Could you check a few things on this model? Use its own coordinates, in mm. A direction names the side the tool comes from. Give positions to 0.01 mm unless a question says otherwise; leave off trailing zeros. Loops run counter-clockwise (first coordinate to the right, second up) from the corner with the lowest first, then second, coordinate; pieces in that order, holes last. Notation, with made-up numbers: (1, 73) - (37, 73) arc R25 cw to (37, 99) - close; hole circle Ø8 at (6.25, 81.25). An arc over 180 degrees is marked (long way). Write each question's results on one line, items separated by ' | '. Start each with the question number.
```python
from build123d import *

# Parameters (mm, degrees)
SKETCH1_R             = 37.5
BOSS_EXTRUDE1_DEPTH   = 10
SKETCH2_R             = 31.5
CUT_EXTRUDE1_DEPTH    = 6.5
SKETCH4_R             = 15.75
BOSS_EXTRUDE2_DEPTH   = 6.5
SKETCH5_R             = 3
CUT_EXTRUDE2_DEPTH    = 3.5
CIRPATTERN3_OUTLINE_R = 3
CIRPATTERN3_DEPTH     = 3.5
BOSS_EXTRUDE3_DEPTH   = 5
CIRPATTERN4_COUNT     = 4
SKETCH9_R             = 4.5
CUT_EXTRUDE3_DEPTH    = 2
CIRPATTERN5_COUNT     = 4
SKETCH10_R            = 1
CUT_EXTRUDE4_DEPTH    = 5
LPATTERN1_COUNT       = 2
LPATTERN1_PITCH       = 174
LPATTERN1_COUNT_DIR2  = 2
LPATTERN1_PITCH_DIR2  = 24
SKETCH11_R            = 2
CUT_EXTRUDE5_DEPTH    = 1
LPATTERN2_COUNT       = 2
LPATTERN2_PITCH       = 174
LPATTERN2_COUNT_DIR2  = 2
LPATTERN2_PITCH_DIR2  = 24


# Read off the part's stored shape, not the designer's step: CirPattern3
with BuildPart() as part:
    # Sketch1 → Boss-Extrude1 (new body)
    with BuildSketch(Plane(origin=(0, 0, 0), x_dir=(1, 0, 0), z_dir=(0, 1, 0))):
        with Locations(Location((0, 0, 0), (0, 0, 270))):
            Circle(SKETCH1_R)
    extrude(amount=BOSS_EXTRUDE1_DEPTH)

    # Sketch2 → Cut-Extrude1 (cut)
    with BuildSketch(Plane(origin=(0, 10, 0), x_dir=(1, 0, 0), z_dir=(0, 1, 0))):
        with Locations(Location((0, 0, 0), (0, 0, 270))):
            Circle(SKETCH2_R)
    extrude(amount=-CUT_EXTRUDE1_DEPTH, mode=Mode.SUBTRACT)

    # Sketch4 → Boss-Extrude2 (add)
    with BuildSketch(Plane(origin=(0, 3.5, 0), x_dir=(1, 0, 0), z_dir=(0, 1, 0))):
        with Locations(Location((0, 0, 0), (0, 0, 90))):
            Circle(SKETCH4_R)
    extrude(amount=BOSS_EXTRUDE2_DEPTH)

    # Sketch5 → Cut-Extrude2 (cut)
    with BuildSketch(Plane.XZ):
        with Locations(Location((0, 25, 0), (0, 0, 270))):
            Circle(SKETCH5_R)
    extrude(amount=-CUT_EXTRUDE2_DEPTH, mode=Mode.SUBTRACT)

    # CirPattern3 outline → CirPattern3 (cut)
    with BuildSketch(Plane(origin=(0, 0, 0), x_dir=(1, 0, 0), z_dir=(0, 1, 0))):
        with Locations((-25, 0)):
            Circle(CIRPATTERN3_OUTLINE_R)
        with Locations((0, 25)):
            Circle(CIRPATTERN3_OUTLINE_R)
        with Locations((25, 0)):
            Circle(CIRPATTERN3_OUTLINE_R)
    extrude(amount=CIRPATTERN3_DEPTH, mode=Mode.SUBTRACT)

    # Sketch7 → Boss-Extrude3 (add)
    with BuildSketch(Plane.XZ):
        with BuildLine():
            Line((34.583232932, 14.5), (92.000000002, 14.5))
            Line((92.000000002, 14.5), (92.000000002, -14.5))
            Line((92.000000002, -14.5), (34.583232932, -14.5))
            ThreePointArc((34.583232932, -14.5), (37.5, 0), (34.583232932, 14.5))
        make_face()
    boss_extrude3 = extrude(amount=-BOSS_EXTRUDE3_DEPTH)

    # CirPattern4: Boss-Extrude3 ×4 about axis, 2 skipped
    cirpattern4_axis = Axis((0, 0, 0), (0, 1, 0))
    add([boss_extrude3.rotate(cirpattern4_axis, i * 360 / CIRPATTERN4_COUNT) for i in range(1, CIRPATTERN4_COUNT) if i not in (1, 3)])

    # Sketch9 → Cut-Extrude3 (cut)
    with BuildSketch(Plane.XZ):
        with Locations(Location((25, 0, 0), (0, 0, 270))):
            Circle(SKETCH9_R)
    cut_extrude3 = extrude(amount=-CUT_EXTRUDE3_DEPTH, mode=Mode.SUBTRACT)

    # CirPattern5: Cut-Extrude3 ×4 about axis
    cirpattern5_axis = Axis((0, 0, 0), (0, 1, 0))
    for i in range(1, CIRPATTERN5_COUNT):
        add(cut_extrude3.rotate(cirpattern5_axis, i * 360 / CIRPATTERN5_COUNT), mode=Mode.SUBTRACT)

    # Sketch10 → Cut-Extrude4 (cut)
    with BuildSketch(Plane(origin=(0, 0, 0), x_dir=(-1, 0, 0), z_dir=(0, -1, 0))):
        with Locations(Location((-87, -12, 0), (0, 0, 90))):
            Circle(SKETCH10_R)
    cut_extrude4 = extrude(amount=-CUT_EXTRUDE4_DEPTH, mode=Mode.SUBTRACT)

    # LPattern1: Cut-Extrude4 2 × 2
    with Locations(*[(-i * LPATTERN1_PITCH, 0, -j * LPATTERN1_PITCH_DIR2) for i in range(LPATTERN1_COUNT) for j in range(LPATTERN1_COUNT_DIR2) if (i, j) != (0, 0)]):
        add(cut_extrude4, mode=Mode.SUBTRACT)

    # Sketch11 → Cut-Extrude5 (cut)
    with BuildSketch(Plane(origin=(0, 5, 0), x_dir=(1, 0, 0), z_dir=(0, 1, 0))):
        with Locations(Location((87, -12, 0), (0, 0, 270))):
            Circle(SKETCH11_R)
    cut_extrude5 = extrude(amount=-CUT_EXTRUDE5_DEPTH, mode=Mode.SUBTRACT)

    # LPattern2: Cut-Extrude5 2 × 2
    with Locations(*[(-i * LPATTERN2_PITCH, 0, -j * LPATTERN2_PITCH_DIR2) for i in range(LPATTERN2_COUNT) for j in range(LPATTERN2_COUNT_DIR2) if (i, j) != (0, 0)]):
        add(cut_extrude5, mode=Mode.SUBTRACT)


solid = part.part
```
Q1. If we mould it in two halves opening along Z, with no side actions, what happens to faces 4 (the face through (-22, 2, 1)), 5 (the face through (0, 10, 0)), 6 (the face through (7.4, 3.5, -14.4)), 7 (the face through (63, 2, 14.5))? For each: +Z half, -Z half, draft (parallel to the pull), parting line (faces both ways), or undercut.
Q2. I need wall thicknesses on L1, parallel to Z at x = -87, y = 1.75; L2, parallel to Z at x = 1, y = 6; L3, parallel to Y at x = -80.5, z = -5.5. Which ranges of each line are inside material? Lowest first, please. Write a range as from..to.
Q3. I want a section at C-C, the plane y = 7. List the corners of the cut face in (x, z) for me, then the cut area to 3 significant figures.
Q4. I want a section at D-D, the plane z = -25. List the corners of the cut face in (x, y) for me.
Q5. I want a section at B-B, the plane x = 0. List the corners of the cut face in (y, z) for me.
Q6. Which directions (+Z, -Z, +X, -X, +Y, -Y) give clear straight access to the entire face, cutting with the end or side of a thin tool? Please do faces 1 (the face through (2.419, 0.986, 28.794)), 2 (the face through (-92, 2, 0)), 3 (the face through (-85.017, 4.507, -12.26)).
Q7. I want a section at A-A, the plane z = 0. State how many separate pieces and enclosed holes the cut face has, then the cut area to 3 significant figures.
Q8. I'm going to push flat-ended pins straight in: pin 1 Ø1 at (y, z) = (1, 24.5) entering from +X; pin 2 Ø1.2 at (x, z) = (87, 11) entering from +Y; pin 3 Ø11.5 at (x, z) = (-25, 0) entering from +Y. Where does each tip first touch, or does it pass through?
Conclusion:
1) face 4: undercut | face 5: draft | face 6: undercut | face 7: +Z half
2) L1: -14.5..-13, -11..11, 13..14.5 | L2: -37.49..-31.48, -15.72..15.72, 31.48..37.49 | L3: 0..5
3) outline: circle Ø75 at (0, 0); circle Ø31.5 at (0, 0); hole circle Ø63 at (0, 0) | area: 2,080 mm^2
4) outline: (-27.95, 0) - (-4.5, 0) - (-4.5, 2) - (-3, 2) - (-3, 3.5) - (-19.16, 3.5) - (-19.16, 10) - (-27.95, 10) - close; (3, 2) - (4.5, 2) - (4.5, 0) - (27.95, 0) - (27.95, 10) - (19.16, 10) - (19.16, 3.5) - (3, 3.5) - close
5) outline: (0, -37.5) - (10, -37.5) - (10, -31.5) - (3.5, -31.5) - (3.5, -28) - (2, -28) - (2, -29.5) - (0, -29.5) - close; (0, -20.5) - (2, -20.5) - (2, -22) - (3.5, -22) - (3.5, -15.75) - (10, -15.75) - (10, 15.75) - (3.5, 15.75) - (3.5, 22) - (2, 22) - (2, 20.5) - (0, 20.5) - close; (0, 29.5) - (2, 29.5) - (2, 28) - (3.5, 28) - (3.5, 31.5) - (10, 31.5) - (10, 37.5) - (0, 37.5) - close
6) face 1: -Y | face 2: +Z, -Z, -X, +Y, -Y | face 3: +Y
7) separate pieces: 3 | enclosed holes: 0 | area: 1,040 mm^2
8) pin 1: x = 28.81 | pin 2: y = 4 | pin 3: y = 3.5
